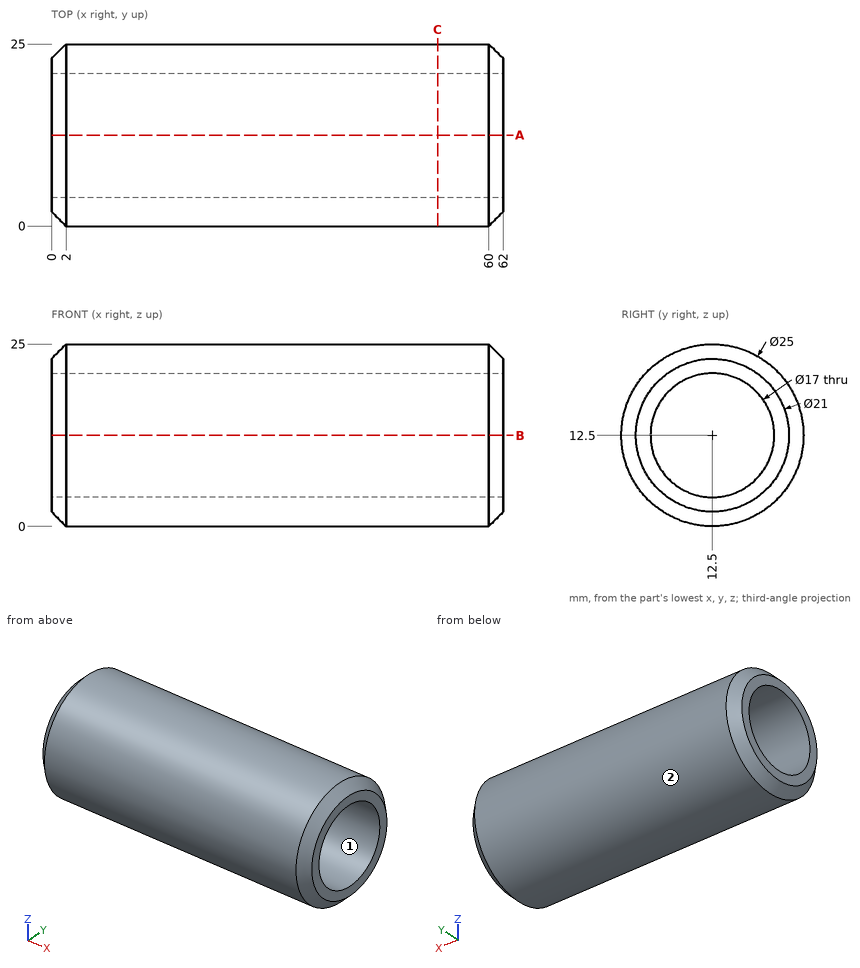
Could you check a few things on this drawing? It's one solid part, dimensions in mm from its lowest x, y, z. Coordinates: 2 decimals unless noted, no trailing zeros. Loops run counter-clockwise (first coordinate to the right, second up) from the corner with the lowest first, then second, coordinate; pieces in that order, holes last.
1. For P1, Ø3, axis at x = 46, y = 10.5, coming from the -Z side; P2, Ø8, axis at x = 51.5, z = 5, coming from the +Y side; P3, Ø8, axis at x = 31, z = 20.5, coming from the +Y side; P4, Ø4, axis at y = 10.5, z = 8, coming from the -X side, each with a flat end and sliding along its axis, tell me the tip position at first contact or that it passes through.
2. Imagine slicing it at A-A (y = 12.5). Please give me the cut outline in (x, z).
3. Imagine slicing it at C-C (x = 53). Please give me the cut outline in (y, z), and give its area (3 significant figures).
4. I need wall thicknesses on L1, parallel to Y at x = 22.5, z = 12.5; L2, parallel to Z at x = 54.5, y = 8; L3, parallel to Z at x = 6.5, y = 18.5. Which ranges of each line are inside material? Lowest first, please.
5. We'd pull the mould along Z, two halves only. Please class the marked faces 1 and 2: released by +Z, released by -Z, zero draft, split by the parting line, or undercut.
Computed values:
1. P1: stops at z = 0.01
1. P2: stops at y = 24.5
1. P3: stops at y = 24.34
1. P4: passes through
2. outline: (0, 2) - (2, 0) - (60, 0) - (62, 2) - (62, 4) - (0, 4) - close; (0, 21) - (62, 21) - (62, 23) - (60, 25) - (2, 25) - (0, 23) - close
3. outline: circle Ø25 at (12.5, 12.5); hole circle Ø17 at (12.5, 12.5)
3. area: 264 mm2
4. L1: y = 0 to 4, 21 to 25
4. L2: z = 0.84 to 5.29, 19.71 to 24.16
4. L3: z = 1.53 to 6.48, 18.52 to 23.47
5. face 1: undercut
5. face 2: split by the parting line
